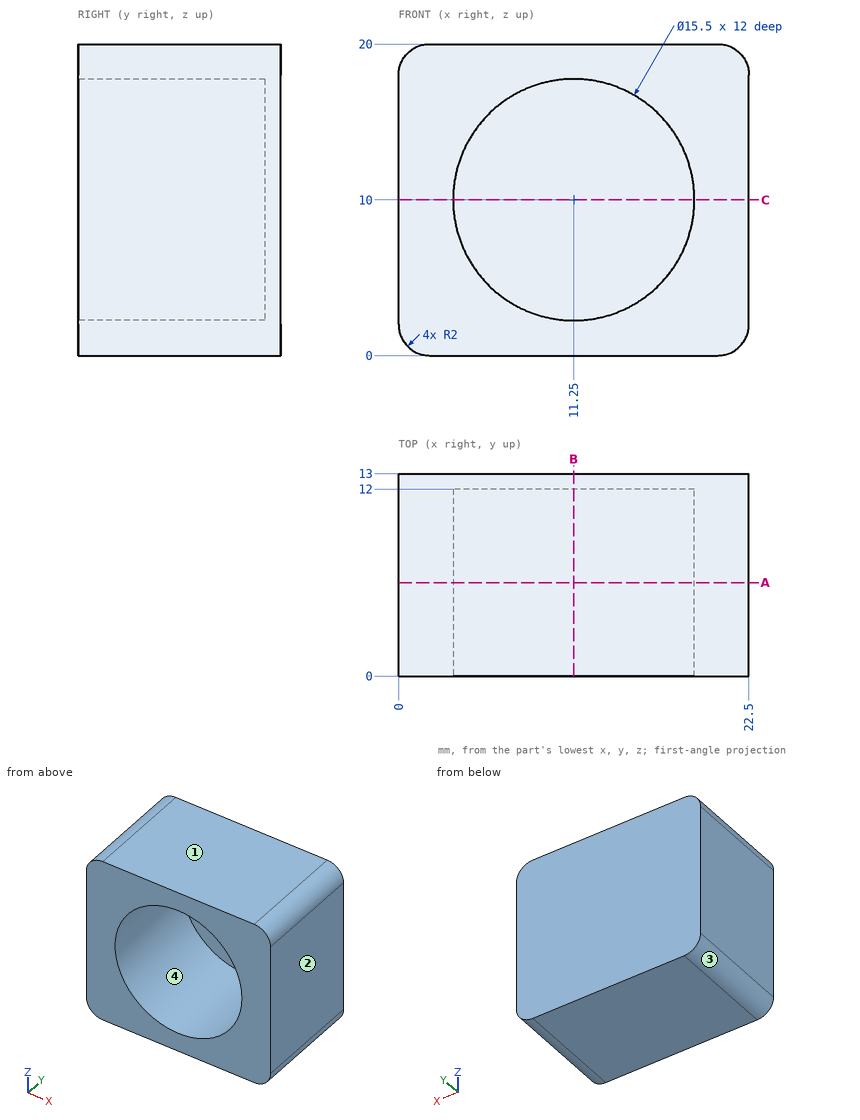
Verification items for this drawing (mm, ordinates from the low corner). Coordinates: 2 decimals unless noted, no trailing zeros. Order: outer loops, then holes, each group sorted by start corner. A loop starts at its lowest first (then second) coordinate and runs counter-clockwise, first axis right, second up. Notation, with made-up numbers: (-35, -33.5) - (-17, -33.5) arc R11 ccw to (-17, -28.5) - close; hole circle Ø3 at (70, -17.5). An arc over 180 degrees is marked (long way). Use one line per item in the form item = value.
1. Section check B-B (x = 11.25). Record the boundary of the cut face in (y, z).
Here are the results:
outline = (0, 0) - (13, 0) - (13, 20) - (0, 20) - (0, 17.75) - (12, 17.75) - (12, 2.25) - (0, 2.25) - close
2. Draft check along X on the marked faces 1, 2, 3 and 4. Enter one of: pulls with the +X half, pulls with the -X half, needs draft (parallel to the pull), parting line crosses it, or undercut.
Here are the results:
face_1 = needs draft
face_2 = pulls with the +X half
face_3 = pulls with the -X half
face_4 = undercut
3. Scan lines: line 1 (Z direction, x = 11.25, y = 7); line 2 (X direction, y = 6, z = 14); line 3 (Y direction, x = 14, z = 5.75). Record each from-to range of solid material in increasing order.
Here are the results:
line_1 = 0 to 2.25, 17.75 to 20
line_2 = 0 to 4.61, 17.89 to 22.5
line_3 = 12 to 13
4. Section check A-A (y = 6). Record the boundary of the cut face in (x, z).
Here are the results:
outline = (0, 2) arc R2 ccw to (2, 0) - (20.5, 0) arc R2 ccw to (22.5, 2) - (22.5, 18) arc R2 ccw to (20.5, 20) - (2, 20) arc R2 ccw to (0, 18) - close; hole circle Ø15.5 at (11.25, 10)
5. Gauge pin test, flat end, axial feed: pin 1 (1 mm diameter, centred on y = 3, z = 4.5, fed in from -X). Record the tip position at first contact, or that the pin passes through.
Here are the results:
pin_1 = 0
6. Section check C-C (z = 10). Record the boundary of the cut face in (x, y).
Here are the results:
outline = (0, 0) - (3.5, 0) - (3.5, 12) - (19, 12) - (19, 0) - (22.5, 0) - (22.5, 13) - (0, 13) - close
